```python
from build123d import *

# Parameters (mm, degrees)
BOSS_EXTRUDE1_DEPTH = 62
CUT_EXTRUDE1_DEPTH  = 106.090437243


with BuildPart() as part:
    # Sketch1 → Boss-Extrude1 (new body)
    with BuildSketch(Plane(origin=(0, 0, 0), x_dir=(1, 0, 0), z_dir=(0, 1, 0))):
        Polygon((-12, 0), (12, 0), (12, 70.583238925), (3.257901851, 84), (-3.257901851, 84), (-12, 70.583238925), align=None)
    extrude(amount=BOSS_EXTRUDE1_DEPTH)

    # Sketch2 → Cut-Revolve4 (revolve, cut)
    with BuildSketch(Plane(origin=(0, 0, 0), x_dir=(0, 0, -1), z_dir=(1, 0, 0))):
        Polygon((48, 55.5), (49.5, 54), (48, 52.5), (48, 46), (37.5, 46), (36, 44.5), (34.5, 46), (24, 46), (24, 39.5), (25.5, 38), (24, 36.5), (24, 30), (13.5, 30), (12, 28.5), (10.5, 30), (-12, 30), (-12, 70), (48, 70), align=None)
    revolve(axis=Axis((0, 0, -89), (0, 1, 0)), mode=Mode.SUBTRACT)

    # Sketch3 → Cut-Extrude1 (cut, through all)
    with BuildSketch(Plane.XY):
        with BuildLine():
            Line((12, 15), (8.601411599, 13.928429193))
            ThreePointArc((8.601411599, 13.928429193), (6.817380703, 14.222973886), (6, 15.835863095))
            Line((6, 15.835863095), (6, 22.164136905))
            ThreePointArc((6, 22.164136905), (6.817380703, 23.777026114), (8.601411599, 24.071570807))
            Line((8.601411599, 24.071570807), (12, 23))
            Line((12, 23), (12, 15))
        make_face()
    extrude(amount=-CUT_EXTRUDE1_DEPTH, mode=Mode.SUBTRACT)


solid = part.part
```
Model file for the job. Use its own axes, mm. A direction names the side the tool comes from. Coordinates: 2 decimals unless noted, no trailing zeros. Loops run counter-clockwise (first coordinate to the right, second up) from the corner with the lowest first, then second, coordinate; pieces in that order, holes last. Notation, with made-up numbers: (-0.75, -23) - (57.25, -23) arc R15 ccw to (57.25, -15) - close; hole circle Ø11 at (68.25, 81). An arc over 180 degrees is marked (long way). Write item = value, one per line. Start each with the question number.
Item 1: Wall check: probe 1 along Z at (x, y) = (-1, 57); probe 2 along Y at (x, z) = (-7, -8); probe 3 along X at (y, z) = (18, -22). Give the ranges that are in metal, low to high. Write a range as [from, to].
Item 2: Pull direction X, two halves, no side cores. Call faces 4 (the face through (0, 43, -24)), 5 (the face through (0, 46, -30)), 6 (the face through (-0.2, 29.1, -11.4)): +X half, -X half, draft (parallel to the pull), parting line (faces both ways), or undercut.
Item 3: Drop flat-ended pins along their axis: pin 1 Ø3 at (x, y) = (-7, 19) entering from -Z; pin 2 Ø3 at (y, z) = (19, -59.5) entering from +X; pin 3 Ø13 at (x, z) = (4.5, -29.5) entering from +Y. Give the stop position or say it passes through.
Item 4: 3-axis set-ups, long thin cutter, end or side, ignore diameter. For faces 1 (the face through (-0.2, 29.4, -12.9)), 2 (the face through (-0.2, 54.4, -49.1)), 3 (the face through (10.32, 14.47, -37.37)): which of +Z, -Z, +X, -X, +Y, -Y reach the whole face in a straight line?
Item 5: Saw through at C-C, the plane y = 9. List the corners of the cut face in (x, z), then the cut area to 3 significant figures.
Item 6: Saw through at A-A, the plane y = 19. List the corners of the cut face in (x, z), then the cut area to 3 significant figures.
Item 7: Saw through at B-B, the plane z = -61. List the corners of the cut face in (x, y), then the cut area to 3 significant figures.
Item 8: Saw through at D-D, the plane z = -32.5. List the corners of the cut face in (x, y), then the cut area to 3 significant figures.
Answers:
q1.probe_1 = [-84, -48.01]
q1.probe_2 = [0, 30]
q1.probe_3 = [-12, 6]
q2.face_4 = parting line
q2.face_5 = draft
q2.face_6 = undercut
q3.pin_1 = -80.56
q3.pin_2 = 6
q3.pin_3 = 46
q4.face_1 = +Y
q4.face_2 = +Z
q4.face_3 = +Z, -Z
q5.outline = (-12, -70.58) - (-3.26, -84) - (3.26, -84) - (12, -70.58) - (12, 0) - (-12, 0) - close
q5.area = 1,900 mm2
q6.outline = (-12, -70.58) - (-3.26, -84) - (3.26, -84) - (6, -79.79) - (6, 0) - (-12, 0) - close
q6.area = 1,450 mm2
q7.outline = (-12, 0) - (12, 0) - (12, 15) - (8.6, 13.93) arc R2 cw to (6, 15.84) - (6, 22.16) arc R2 cw to (8.6, 24.07) - (12, 23) - (12, 62) - (-12, 62) - close
q7.area = 1,430 mm2
q8.outline = (-12, 0) - (12, 0) - (12, 15) - (8.6, 13.93) arc R2 cw to (6, 15.84) - (6, 22.16) arc R2 cw to (8.6, 24.07) - (12, 23) - (12, 46) - (-12, 46) - close
q8.area = 1,050 mm2
